from build123d import *

# Parameters (mm, degrees)
SKETCH2_R             = 11
BOSS_EXTRUDE1_DEPTH   = 12.5
SKETCH2_R_2           = 12
SKETCH2_R_3           = 6
BOSS_EXTRUDE1_2_DEPTH = 12.5
BOSS_EXTRUDE2_DEPTH   = 5
BOSS_EXTRUDE3_DEPTH   = 2.5


with BuildPart() as part:
    # Sketch2 → Boss-Extrude1 (new, symmetric)
    with BuildSketch(Plane(origin=(0, 0, 0), x_dir=(1, 0, 0), z_dir=(0, 1, 0))):
        with BuildLine():
            ThreePointArc((-33.466351399, 21), (-54.466351399, 0), (-33.466351399, -21))
            Line((-33.466351399, -21), (-29.307935557, -20.584158416))
            ThreePointArc((-29.307935557, -20.584158416), (-17.213248116, -13.297993595), (-12.466351399, 0))
            ThreePointArc((-12.466351399, 0), (-17.213248116, 13.297993595), (-29.307935557, 20.584158416))
            Line((-29.307935557, 20.584158416), (-33.466351399, 21))
        make_face()
        with Locations(Location((-33.466351399, 0, 0), (0, 0, 270))):
            Circle(SKETCH2_R, mode=Mode.SUBTRACT)
    extrude(amount=BOSS_EXTRUDE1_DEPTH, both=True)



with BuildPart() as body_2:
    # Sketch2 → Boss-Extrude1 2 (new, symmetric)
    with BuildSketch(Plane(origin=(0, 0, 0), x_dir=(1, 0, 0), z_dir=(0, 1, 0))):
        with Locations(Location((56.533648601, 0, 0), (0, 0, 270))):
            Circle(SKETCH2_R_2)
        with Locations(Location((56.533648601, 0, 0), (0, 0, 270))):
            Circle(SKETCH2_R_3, mode=Mode.SUBTRACT)
    extrude(amount=BOSS_EXTRUDE1_2_DEPTH, both=True)


with BuildPart() as part_1:
    add(part.part)

    add(body_2.part)  # Boss-Extrude2 merges body 2
    # Sketch2_3 → Boss-Extrude2 (add, symmetric)
    with BuildSketch(Plane(origin=(0, 0, 0), x_dir=(1, 0, 0), z_dir=(0, 1, 0))):
        with BuildLine():
            ThreePointArc((-12.466351399, 0), (-17.213248116, -13.297993595), (-29.307935557, -20.584158416))
            Line((-29.307935557, -20.584158416), (56.533648601, -12))
            ThreePointArc((56.533648601, -12), (44.533648601, 0), (56.533648601, 12))
            Line((56.533648601, 12), (-29.307935557, 20.584158416))
            ThreePointArc((-29.307935557, 20.584158416), (-17.213248116, 13.297993595), (-12.466351399, 0))
        make_face()
        with BuildLine():
            ThreePointArc((-10.635434162, 10.185736013), (-10.327887019, 13.164322574), (-7.597212937, 14.393135905))
            Line((-7.597212937, 14.393135905), (40.416577367, 9.591756875))
            ThreePointArc((40.416577367, 9.591756875), (41.955623351, 8.591212838), (42.030467559, 6.757051106))
            ThreePointArc((42.030467559, 6.757051106), (40.533648601, 0), (42.030467559, -6.757051106))
            ThreePointArc((42.030467559, -6.757051106), (41.955623351, -8.591212838), (40.416577367, -9.591756875))
            Line((40.416577367, -9.591756875), (-7.597212937, -14.393135905))
            ThreePointArc((-7.597212937, -14.393135905), (-10.327887019, -13.164322574), (-10.635434162, -10.185736013))
            ThreePointArc((-10.635434162, -10.185736013), (-8.466351399, 0), (-10.635434162, 10.185736013))
        make_face(mode=Mode.SUBTRACT)
    extrude(amount=BOSS_EXTRUDE2_DEPTH, both=True)

    # Sketch2_4 → Boss-Extrude3 (add, symmetric)
    with BuildSketch(Plane(origin=(0, 0, 0), x_dir=(1, 0, 0), z_dir=(0, 1, 0))):
        with BuildLine():
            Line((-7.597212937, 14.393135905), (40.416577367, 9.591756875))
            ThreePointArc((40.416577367, 9.591756875), (41.955623351, 8.591212838), (42.030467559, 6.757051106))
            ThreePointArc((42.030467559, 6.757051106), (40.533648601, 0), (42.030467559, -6.757051106))
            ThreePointArc((42.030467559, -6.757051106), (41.955623351, -8.591212838), (40.416577367, -9.591756875))
            Line((40.416577367, -9.591756875), (-7.597212937, -14.393135905))
            ThreePointArc((-7.597212937, -14.393135905), (-10.327887019, -13.164322574), (-10.635434162, -10.185736013))
            ThreePointArc((-10.635434162, -10.185736013), (-8.466351399, 0), (-10.635434162, 10.185736013))
            ThreePointArc((-10.635434162, 10.185736013), (-10.327887019, 13.164322574), (-7.597212937, 14.393135905))
        make_face()
    extrude(amount=BOSS_EXTRUDE3_DEPTH, both=True)


solid = part_1.part
Verification items for the finished model (mm, model axes). A direction names the side the tool comes from. Give positions to 0.01 mm unless a question says otherwise; leave off trailing zeros. Loops run counter-clockwise (first coordinate to the right, second up) from the corner with the lowest first, then second, coordinate; pieces in that order, holes last.
1) Depth check by flat-ended pin: pin 1 Ø1.5 at (y, z) = (-6.5, 8.5) entering from +X; pin 2 Ø5 at (x, y) = (-24, 2) entering from +Z; pin 3 Ø10 at (y, z) = (-5.5, -11.5) entering from +X. Enter the tip coordinate at first touch or a pass-through.
2) Sectioned sample at D-D, the plane x = -26. Enter the section's corners in (y, z), then the cut area to 3 significant figures.
3) Draft check along Z on faces 1 (the cylindrical face through (-26.032, -0.175, -8.107)), 2 (the cylindrical face through (-10.35, -3.73, -13.13)), 3 (the flat face through (54, 12.5, -6)). Enter one of: pulls with the +Z half, pulls with the -Z half, needs draft (parallel to the pull), parting line crosses it, or undercut.
4) Thickness scan on line 1 along X through (y, z) = (-5.25, 0); line 2 along X through (y, z) = (1.25, 0); line 3 along X through (y, z) = (-7, -0.5). Record the ranges inside material, lowest first.
5) Sectioned sample at B-B, the plane y = -0.5. Enter the section's corners in (x, z).
6) Sectioned sample at C-C, the plane z = -2.5. Enter the section's corners in (x, y), then the cut area to 3 significant figures.
7) Set-up check for faces 4 (the cylindrical face through (41.969, -3.732, 8.568)), 5 (the cylindrical face through (62.483, -0.175, -0.781)), 6 (the flat face through (16, 2.5, 0)): record each of +Z, -Z, +X, -X, +Y, -Y from which the full face is reachable in a straight line by a thin tool's end or side.
8) Sectioned sample at A-A, the plane y = 10.5. Enter the section's corners in (x, z).
Answers:
1. pin 1: stops at x = 65.7
1. pin 2: stops at z = 20.3
1. pin 3: stops at x = 66.62
2. outline: (-12.5, -19.63) - (-5, -19.63) - (-5, -20.25) - (5, -20.25) - (5, -19.63) - (12.5, -19.63) - (12.5, -8.08) - (-12.5, -8.08) - close; (-12.5, 8.08) - (12.5, 8.08) - (12.5, 19.63) - (5, 19.63) - (5, 20.25) - (-5, 20.25) - (-5, 19.63) - (-12.5, 19.63) - close
2. area: 590 mm2
3. face 1: undercut
3. face 2: undercut
3. face 3: needs draft
4. line 1: x = -54.47 to -44.47, -22.47 to -12.47, 44.53 to 50.53, 62.53 to 68.53
4. line 2: x = -54.47 to -44.47, -22.47 to 50.53, 62.53 to 68.53
4. line 3: x = -54.46 to -44.45, -22.48 to -12.47, 44.54 to 50.55, 62.51 to 68.52
5. outline: (-33.47, -21) - (56.53, -12) arc R12 ccw to (56.53, 12) - (-33.47, 21) arc R21 ccw to start; hole circle Ø22 at (-33.47, 0); hole circle Ø12 at (56.53, 0)
6. outline: (-54.32, -12.5) - (-44.18, -12.5) - (-44.18, 12.5) - (-54.32, 12.5) - close; (-22.75, -12.5) - (-12.62, -12.5) - (-12.62, -5) - (-8.59, -5) - (-8.59, -2.5) - (40.73, -2.5) - (40.73, -5) - (44.8, -5) - (44.8, -12.5) - (51.08, -12.5) - (51.08, 12.5) - (44.8, 12.5) - (44.8, 5) - (40.73, 5) - (40.73, 2.5) - (-8.59, 2.5) - (-8.59, 5) - (-12.62, 5) - (-12.62, 12.5) - (-22.75, 12.5) - close; (61.99, -12.5) - (68.27, -12.5) - (68.27, 12.5) - (61.99, 12.5) - close
6. area: 1,150 mm2
7. face 4: -Y
7. face 5: +Y, -Y
7. face 6: +Y
8. outline: (-33.47, -21) - (-29.31, -20.58) arc R21 ccw to (-29.31, 20.58) - (-33.47, 21) arc R21 ccw to start; circle Ø24 at (56.53, 0); hole circle Ø22 at (-33.47, 0); hole circle Ø12 at (56.53, 0)
